Part model, mm, in its own coordinate system. Face numbers are marked on the shaded views. Give positions to 0.01 mm unless a question says otherwise; leave off trailing zeros. Write each loop counter-clockwise with the first axis right and the second up, starting at its lowest first coordinate (ties: lowest second). Pieces come first, ordered by that corner, then holes. Notation, with made-up numbers: M -40,-35.5 L -27,-35.5 A4 ccw -27,-29.5 Z; hole C -14.75,65 d3. An arc over 180 degrees is marked long. Answer as CSV lines item,"result". Start each with the question number.
Item 1: Wall check: L1, parallel to X at y = 41.5, z = 6.25; L2, parallel to Z at x = 124, y = 30; L3, parallel to Z at x = 46.5, y = 30. Give the ranges that are in metal, low to high. Write a range as from..to.
Item 2: Band-saw the part on B-B, the plane x = 133.5. List the corners of the cut face in (y, z).
Item 3: Band-saw the part on A-A, the plane x = 32. List the corners of the cut face in (y, z), then the cut area to 3 significant figures.
Item 4: Two-plate mould, pull along X, no slides. Class the marked faces 1, 2 and 3: +X half, -X half, draft (parallel to the pull), parting line (faces both ways), or undercut.
Item 5: Pin check, flat tips, straight feed: pin 1 (3 mm diameter, centred on y = 39, z = 10.5, fed in from +X); pin 2 (8 mm diameter, centred on x = -63, y = 25.5, fed in from +Z); pin 3 (3 mm diameter, centred on x = -70.5, y = 8.5, fed in from +Z). Stop position of each tip, or through.
Item 6: Band-saw the part on C-C, the plane x = -70.5. List the corners of the cut face in (y, z), then the cut area to 3 significant figures.
from build123d import *

# Parameters (mm, degrees)
SKETCH037_W      = 2
SKETCH037_H      = 37
EXTRUDE036_DEPTH = 1
FILLET012_R      = 0.25
SKETCH038_W      = 13.25
SKETCH038_H      = 36
EXTRUDE037_DEPTH = 2
SKETCH031_W      = 37
SKETCH031_H      = 2.5
EXTRUDE029_DEPTH = 120
SKETCH030_W      = 56
SKETCH030_H      = 13.5
EXTRUDE028_DEPTH = 41
SKETCH036_W      = 120
SKETCH036_H      = 8
EXTRUDE035_DEPTH = 2
FILLET011_R      = 1
FILLET013_R      = 4
FILLET014_R      = 1


with BuildPart() as velcrobands:
    # Sketch037 → Extrude036 (new body)
    with BuildSketch(Plane.XY.offset(5.5)):
        with Locations((174, 26.5)):
            Rectangle(SKETCH037_W, SKETCH037_H)
        with Locations((147, 26.5)):
            Rectangle(SKETCH037_W, SKETCH037_H)
    extrude(amount=EXTRUDE036_DEPTH)

    # Fillet012
    fillet012_edges = [velcrobands.edges().sort_by_distance(p)[0] for p in [
        (148, 26.5, 6.5),
        (146, 26.5, 6.5),
        (173, 26.5, 6.5),
        (175, 26.5, 6.5),
    ]]
    fillet(fillet012_edges, radius=FILLET012_R)


with BuildPart() as sensorcuts:
    # Sketch038 → Extrude037 (new body)
    with BuildSketch(Plane.XY.offset(-0.75)):
        with Locations((151.375, 26.5)):
            Rectangle(SKETCH038_W, SKETCH038_H)
    extrude(amount=-EXTRUDE037_DEPTH)


with BuildPart() as extrude029:
    # Sketch031 → Extrude029 (new body)
    with BuildSketch(Plane.YZ.offset(56)):
        with Locations((26.412533, 0.5)):
            Rectangle(SKETCH031_W, SKETCH031_H)
    extrude(amount=EXTRUDE029_DEPTH)


with BuildPart() as band002:
    # Sketch030 → Extrude028 (new body)
    with BuildSketch(Plane.XZ.offset(-6)):
        Polygon((175, 5.5), (60, 5.5), (60, 17.5), (-4, 17.5), (-4, 2.5), (-122, 2.5), (-122, -2.5), (175, -2.5), align=None)
        with Locations((28, 6.75)):
            Rectangle(SKETCH030_W, SKETCH030_H, mode=Mode.SUBTRACT)
    extrude(amount=-EXTRUDE028_DEPTH)

    # Cut002: cut Extrude029
    add(extrude029.part, mode=Mode.SUBTRACT)

    # Cut005: cut sensorCuts
    add(sensorcuts.part, mode=Mode.SUBTRACT)


with BuildPart() as fillet014:
    # Sketch036 → Extrude035 (new body)
    with BuildSketch(Plane.XY.offset(2.5)):
        with Locations((-62, 43)):
            Rectangle(SKETCH036_W, SKETCH036_H)
        with Locations((-62, 10)):
            Rectangle(SKETCH036_W, SKETCH036_H)
    extrude(amount=EXTRUDE035_DEPTH)

    # Fillet011
    fillet011_edges = [fillet014.edges().sort_by_distance(p)[0] for p in [
        (-62, 14, 4.5),
        (-62, 6, 4.5),
        (-62, 47, 4.5),
        (-62, 39, 4.5),
    ]]
    fillet(fillet011_edges, radius=FILLET011_R)

    # Fusion011: union velcroBands, band002
    add(velcrobands.part)
    add(band002.part)

    # Fillet013
    fillet013_edges = [fillet014.edges().sort_by_distance(p)[0] for p in [
        (60, 26.5, 17.5),
        (-4, 26.5, 17.5),
        (0, 26.5, 0),
        (0, 26.5, 13.5),
        (56, 26.5, 13.5),
    ]]
    fillet(fillet013_edges, radius=FILLET013_R)

    # Fillet014
    fillet014_edges = [fillet014.edges().sort_by_distance(p)[0] for p in [
        (26.5, 6, -2.5),
        (28, 6, 13.5),
        (26.5, 47, -2.5),
        (28, 47, 13.5),
        (56, 26.412533, 1.75),
    ]]
    fillet(fillet014_edges, radius=FILLET014_R)


solid = fillet014.part
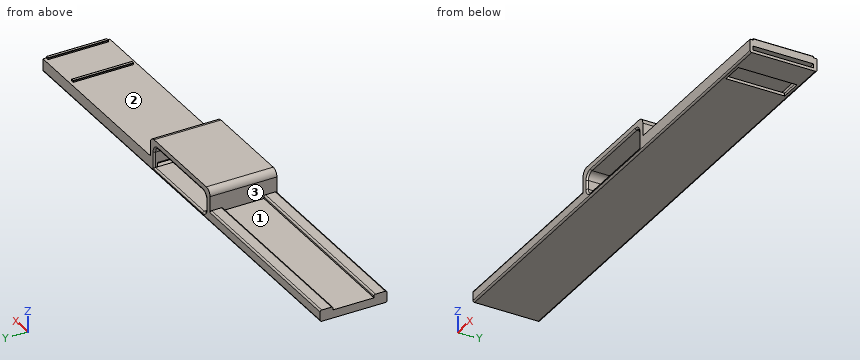
Output:
1,L1,"-4..0, 56..60, 146..148, 173..175"
1,L2,"-2.5..-0.75, 1.75..5.5"
1,L3,"-2.5..0, 13.5..17.5"
2,outline,"M 6,-1.5 A1 ccw 7,-2.5 L 46,-2.5 A1 ccw 47,-1.5 L 47,5.5 L 6,5.5 Z; hole M 7.91,-0.75 L 44.91,-0.75 L 44.91,1.75 L 7.91,1.75 Z"
3,outline,"M 6,-1.5 A1 ccw 7,-2.5 L 46,-2.5 A1 ccw 47,-1.5 L 47,-1 A1 ccw 46,0 L 7,0 A1 ccw 6,-1 Z; M 6,14.5 A1 ccw 7,13.5 L 46,13.5 A1 ccw 47,14.5 L 47,17.5 L 6,17.5 Z"
3,area,"265 mm²"
4,face 1,"draft"
4,face 2,"undercut"
4,face 3,"-X half"
5,pin 1,"x = 60"
5,pin 2,"z = 2.5"
5,pin 3,"z = 4.5"
6,outline,"M 6,-1.5 A1 ccw 7,-2.5 L 46,-2.5 A1 ccw 47,-1.5 L 47,3.5 A1 ccw 46,4.5 L 40,4.5 A1 ccw 39,3.5 L 39,2.5 L 14,2.5 L 14,3.5 A1 ccw 13,4.5 L 7,4.5 A1 ccw 6,3.5 Z"
6,area,"236 mm²"
